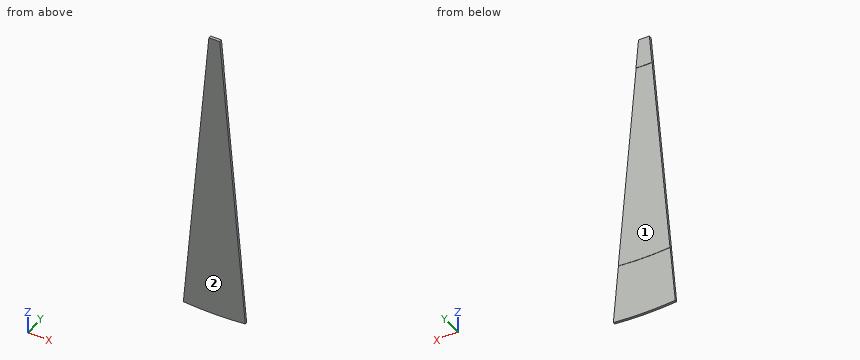
```python
from build123d import *

# Parameters (mm, degrees)
EXTRUSION1_DEPTH = 10
EXTRUSION2_DEPTH = 9
EXTRUSION3_DEPTH = 8


with BuildPart() as part:
    # Esquisse1 → Extrusion1 (new body)
    with BuildSketch(Plane(origin=(0, 0, 0), x_dir=(1, 0, 0), z_dir=(0, 1, 0))):
        with BuildLine():
            Line((18.5, 0), (-18.5, 0))
            Line((-18.5, 0), (-27.145176189, 98.814816012))
            ThreePointArc((-27.145176189, 98.814816012), (0, 100), (27.145176189, 98.814816012))
            Line((27.145176189, 98.814816012), (18.5, 0))
        make_face()
    extrude(amount=EXTRUSION1_DEPTH)

    # Esquisse2 → Extrusion2 (add)
    with BuildSketch(Plane.XZ):
        with BuildLine():
            Line((-27.145176189, -98.814816012), (-88.154196113, -796.151104676))
            ThreePointArc((-88.154196113, -796.151104676), (0, -800), (88.154196113, -796.151104676))
            Line((88.154196113, -796.151104676), (27.145176189, -98.814816012))
            ThreePointArc((27.145176189, -98.814816012), (0, -100), (-27.145176189, -98.814816012))
        make_face()
    extrude(amount=-EXTRUSION2_DEPTH)

    # Esquisse5 → Extrusion3 (add)
    with BuildSketch(Plane.XZ):
        with BuildLine():
            Line((-88.154196113, -796.151104676), (-105.585344662, -995.390044295))
            ThreePointArc((-105.585344662, -995.390044295), (0, -1000), (105.585344662, -995.390044295))
            Line((105.585344662, -995.390044295), (88.154196113, -796.151104676))
            ThreePointArc((88.154196113, -796.151104676), (0, -800), (-88.154196113, -796.151104676))
        make_face()
    extrude(amount=-EXTRUSION3_DEPTH)


solid = part.part
```
Input: part model. Units: mm. Frame: model coordinates. Face numbers are marked on the shaded views. A direction names the side the tool comes from. Coordinates: 2 decimals unless noted, no trailing zeros. Loops run counter-clockwise (first coordinate to the right, second up) from the corner with the lowest first, then second, coordinate; pieces in that order, holes last. Notation, with made-up numbers: M -23,26.25 L 36,26.25 A7 ccw 36,31.25 Z; hole C -15,-32 d3. An arc over 180 degrees is marked long. Answer in a Markdown table with one row per item.
1. Section B-B, the plane x = 10. Output: boundary loops of the cut face in (y, z).
Response:
| item | result |
|---|---|
| outline | M 0,-999.96 L 8,-999.96 L 8,-799.95 L 9,-799.95 L 9,-99.84 L 10,-99.84 L 10,0 L 0,0 Z |
2. First-contact query: pin 1 (1.5 mm diameter, centred on y = 7, z = -850.5, fed in from -X); pin 2 (4 mm diameter, centred on x = -43.5, z = -654.5, fed in from +Y); pin 3 (6 mm diameter, centred on y = 7.5, z = -722.5, fed in from +X). Flat tips, straight axial feed; report the tip coordinate or a pass-through.
Response:
| item | result |
|---|---|
| pin 1 | stops at x = -92.97 |
| pin 2 | stops at y = 9 |
| pin 3 | stops at x = 81.97 |
3. Section D-D, the plane x = -36. Output: boundary loops of the cut face in (y, z).
Response:
| item | result |
|---|---|
| outline | M 0,-999.46 L 8,-999.46 L 8,-799.36 L 9,-799.36 L 9,-200.03 L 0,-200.03 Z |
4. Section A-A, the plane y = 2.25. Output: boundary loops of the cut face in (x, z).
Response:
| item | result |
|---|---|
| outline | M -105.59,-995.39 A1211.46 ccw 105.59,-995.39 L 18.5,0 L -18.5,0 Z |
5. Section C-C, the plane z = -491. Output: boundary loops of the cut face in (x, y), then the cut area to 3 significant figures.
Response:
| item | result |
|---|---|
| outline | M -61.46,0 L 61.46,0 L 61.46,9 L -61.46,9 Z |
| area | 1,110 mm2 |
6. Material intervals for line 1 (Y direction, x = -60, z = -743); line 2 (Y direction, x = 8, z = -857); line 3 (X direction, y = 4.5, z = -478.5), sorted ascending.
Response:
| item | result |
|---|---|
| line 1 | y = 0 to 9 |
| line 2 | y = 0 to 8 |
| line 3 | x = -60.36 to 60.36 |
7. Reachability of the marked faces 1 and 2 from +Z, -Z, +X, -X, +Y, -Y: full face, straight path, thin tool, end or side. Return the list, or none.
Response:
| item | result |
|---|---|
| face 1 | -Z, +X, -X, +Y |
| face 2 | +Z, -Z, +X, -X, -Y |
